For this review, take the finished solid that the model builds, in its own axes (mm). A direction names the side the tool comes from. Coordinates: 2 decimals unless noted, no trailing zeros. Order: outer loops, then holes, each group sorted by start corner. A loop starts at its lowest first (then second) coordinate and runs counter-clockwise, first axis right, second up.
from build123d import *

# Parameters (mm, degrees)
CYLINDER2800_R     = 1.5
CYLINDER2800_DEPTH = 60
CYLINDER2801_R     = 1.5
CYLINDER2801_DEPTH = 60
CYLINDER2802_R     = 1.5
CYLINDER2802_DEPTH = 60
CYLINDER2799_R     = 1.5
CYLINDER2799_DEPTH = 60
BOX1001_W          = 42
BOX1001_H          = 46
BOX1001_DEPTH      = 50
BOX1000_W          = 54
BOX1000_H          = 58
BOX1000_DEPTH      = 9
CHAMFER146_SIZE    = 3


with BuildPart() as obj1:
    # Cylinder2800 → Cylinder2800 (new body)
    with BuildSketch(Plane(origin=(-24, 73, -80), x_dir=(1, 0, 0), z_dir=(0, 0, 1))):
        Circle(CYLINDER2800_R)
    extrude(amount=CYLINDER2800_DEPTH)


with BuildPart() as obj2:
    # Cylinder2801 → Cylinder2801 (new body)
    with BuildSketch(Plane(origin=(-15, 125, -80), x_dir=(1, 0, 0), z_dir=(0, 0, 1))):
        Circle(CYLINDER2801_R)
    extrude(amount=CYLINDER2801_DEPTH)


with BuildPart() as obj3:
    # Cylinder2802 → Cylinder2802 (new body)
    with BuildSketch(Plane(origin=(15, 125, -80), x_dir=(1, 0, 0), z_dir=(0, 0, 1))):
        Circle(CYLINDER2802_R)
    extrude(amount=CYLINDER2802_DEPTH)


with BuildPart() as compound1251:
    # Cylinder2799 → Cylinder2799 (new body)
    with BuildSketch(Plane(origin=(24, 73, -80), x_dir=(1, 0, 0), z_dir=(0, 0, 1))):
        Circle(CYLINDER2799_R)
    extrude(amount=CYLINDER2799_DEPTH)

    # Compound1251: union obj1, obj2, obj3
    add(obj1.part)
    add(obj2.part)
    add(obj3.part)


with BuildPart() as compound1251_1:
    # Compound1251 placement: moved
    add(compound1251.part.moved(Location((0, 0, 120))))


with BuildPart() as krychle1000:
    # Box1001 → Box1001 (new body)
    with BuildSketch(Plane(origin=(-21, 76, 38), x_dir=(1, 0, 0), z_dir=(0, 0, 1))):
        with Locations((21, 23)):
            Rectangle(BOX1001_W, BOX1001_H)
    extrude(amount=BOX1001_DEPTH)


with BuildPart() as cut1063:
    # Box1000 → Box1000 (new body)
    with BuildSketch(Plane(origin=(-27, 70, 75), x_dir=(1, 0, 0), z_dir=(0, 0, 1))):
        with Locations((27, 29)):
            Rectangle(BOX1000_W, BOX1000_H)
    extrude(amount=BOX1000_DEPTH)

    # Cut1068: cut Krychle1000
    add(krychle1000.part, mode=Mode.SUBTRACT)


with BuildPart() as cut1063_1:
    # Cut1068 placement: moved
    add(cut1063.part.moved(Location((0, 0, 10))))

    # Chamfer146
    chamfer146_edges = [cut1063_1.edges().sort_by_distance(p)[0] for p in [
        (-27, 128, 89.5),
        (27, 128, 89.5),
    ]]
    chamfer(chamfer146_edges, length=CHAMFER146_SIZE)

    # Cut1063: cut Compound1251
    add(compound1251_1.part, mode=Mode.SUBTRACT)


solid = cut1063_1.part
1. To check wall thickness, follow L1, parallel to Y at x = -15, z = 89.75; L2, parallel to X at y = 73, z = 87.5; L3, parallel to X at y = 125, z = 87.5. State the ranges of each line that lie inside material, in increasing order.
Answer below:
L1: y = 70 to 76, 122 to 123.5, 126.5 to 128
L2: x = -27 to -25.5, -22.5 to 22.5, 25.5 to 27
L3: x = -27 to -16.5, -13.5 to 13.5, 16.5 to 27
2. Clearance check with flat-ended pins moving along their axes: pin 1 Ø3.5 at (x, y) = (24, 73) entering from -Z; pin 2 Ø2.5 at (x, y) = (-15, 125) entering from +Z. State where each tip first meets the part, or that it passes through.
Answer below:
pin 1: stops at z = 85
pin 2: passes through
3. Machinability: for faces 1 (the face through (0, 122, 89)), 2 (the face through (27, 97, 89)), which of the approach directions +Z, -Z, +X, -X, +Y, -Y give a long, thin tool a straight path to every point of the face, cutting with its end or side? Answer none if there is none.
Answer below:
face 1: +Z, -Z
face 2: +Z, -Z, +X, +Y, -Y
4. Take a section at A-A, the plane y = 73. Give the boundary of the cut face in (x, z), plus the area to 3 significant figures.
Answer below:
outline: (-27, 85) - (-25.5, 85) - (-25.5, 94) - (-27, 94) - close; (-22.5, 85) - (22.5, 85) - (22.5, 94) - (-22.5, 94) - close; (25.5, 85) - (27, 85) - (27, 94) - (25.5, 94) - close
area: 432 mm2
5. Take a section at B-B, the plane x = 15. Give the boundary of the cut face in (y, z).
Answer below:
outline: (70, 85) - (76, 85) - (76, 94) - (70, 94) - close; (122, 85) - (123.5, 85) - (123.5, 94) - (122, 94) - close; (126.5, 85) - (128, 85) - (128, 94) - (126.5, 94) - close
6. The part is to be moulded in two halves that separate along Y. For faces 3 (the face through (-25, 127, 89)), 4 (the face through (0, 125, 94)), 5 (the face through (21, 99, 89)), say which applies: +Y half, -Y half, draft (parallel to the pull), parting line (faces both ways), or undercut.
Answer below:
face 3: +Y half
face 4: draft
face 5: undercut
7. Take a section at C-C, the plane z = 86.5. Give the boundary of the cut face in (x, y), plus the area to 3 significant figures.
Answer below:
outline: (-27, 70) - (27, 70) - (27, 125) - (24, 128) - (-24, 128) - (-27, 125) - close; hole circle Ø3 at (-24, 73); hole (-21, 76) - (21, 76) - (21, 122) - (-21, 122) - close; hole circle Ø3 at (-15, 125); hole circle Ø3 at (15, 125); hole circle Ø3 at (24, 73)
area: 1,160 mm2
